Autodesk Inventor part; units mm, degrees
ref_plane "YZ Plane" through (0, 0, 0) normal (1, 0, 0) x (0, 1, 0)
ref_plane "XZ Plane" through (0, 0, 0) normal (0, 1, 0) x (-1, 0, 0)
ref_plane "XY Plane" through (0, 0, 0) normal (0, 0, 1) x (1, 0, 0)
sketch "Sketch1" plane through (0, 0, 0) normal (0, 0, 1) x (1, 0, 0)
  circle A0 centre (0, 0) radius 18
  dimension "d0" = 36
extrude "Extrusion1" add sketch "Sketch1" along normal blind 2.5
sketch "Sketch2" plane through (0, 0, 2.5) normal (0, 0, 1) x (1, 0, 0)
  line L0 (0, 0) -> (0, 11)
  circle A0 centre (0, 11) radius 1.25
  circle A1 centre (0, 0) radius 5
  circle A2 centre (7.7782, 7.7782) radius 1.25
  circle A3 centre (11, 0) radius 1.25
  circle A4 centre (7.7782, -7.7782) radius 1.25
  circle A5 centre (0, -11) radius 1.25
  circle A6 centre (-7.7782, -7.7782) radius 1.25
  circle A7 centre (-11, 0) radius 1.25
  circle A8 centre (-7.7782, 7.7782) radius 1.25
  dimension "d3" = 11
  dimension "d4" = 2.5
  dimension "d5" = 10
  dimension "d8" = 360
extrude "Extrusion2" cut sketch "Sketch2" against normal through all
sketch "Sketch3" plane through (0, 0, 2.5) normal (0, 0, 1) x (1, 0, 0)
  circle A0 centre (0, 0) radius 5.25
  dimension "d12" = 10.5
extrude "Extrusion3" cut sketch "Sketch3" against normal through all
sketch "Sketch4" plane through (0, 0, 2.5) normal (0, 0, 1) x (1, 0, 0)
  circle A0 centre (0, 11) radius 1.25
  circle A1 centre (0, 11) radius 1.35
  circle A2 centre (7.7782, 7.7782) radius 1.25
  circle A3 centre (7.7782, 7.7782) radius 1.35
  circle A4 centre (11, 0) radius 1.25
  circle A5 centre (11, 0) radius 1.35
  circle A6 centre (-7.7782, 7.7782) radius 1.25
  circle A7 centre (-7.7782, 7.7782) radius 1.35
  circle A8 centre (-11, 0) radius 1.25
  circle A9 centre (-11, 0) radius 1.35
  circle A10 centre (-7.7782, -7.7782) radius 1.25
  circle A11 centre (-7.7782, -7.7782) radius 1.35
  circle A12 centre (0, -11) radius 1.25
  circle A13 centre (0, -11) radius 1.35
  circle A14 centre (7.7782, -7.7782) radius 1.25
  circle A15 centre (7.7782, -7.7782) radius 1.35
  point P0 (0, 0)
  dimension "d15" = 2.7
  dimension "d16" = 2.7
  dimension "d17" = 2.7
  dimension "d18" = 2.7
  dimension "d19" = 2.7
  dimension "d20" = 2.7
  dimension "d21" = 2.7
  dimension "d22" = 2.7
extrude "Extrusion4" cut sketch "Sketch4" against normal blind 10
properties part number "Pulley_base"
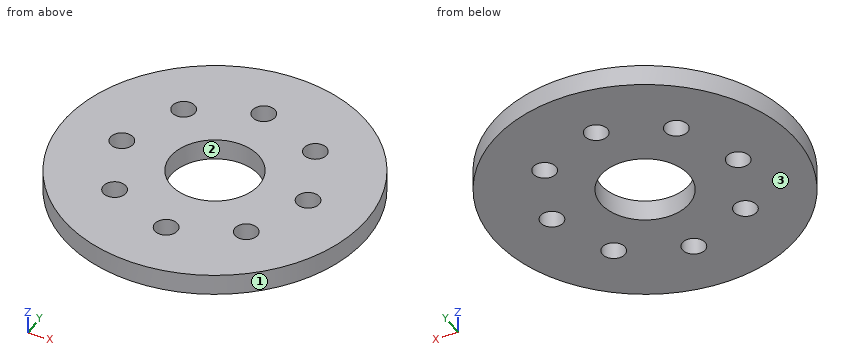
Part model, mm, in its own coordinate system. Face numbers are marked on the shaded views. Round coordinates to 2 decimals unless told otherwise and drop trailing zeros. Loops run counter-clockwise (first coordinate to the right, second up) from the corner with the lowest first, then second, coordinate; pieces in that order, holes last. Notation, with made-up numbers: (58.5, 15.25) -> (114.5, 15.25) arc R23 ccw to (114.5, 38.25) -> close; hole circle Ø8 at (-12, 7.5). An arc over 180 degrees is marked (long way). Use CSV: the item, a comma, the result in double quotes. Start each with the question number.
1) Drop flat-ended pins along their axis: P1, Ø1.5, axis at y = 5.5, z = 0.5, coming from the -X side; P2, Ø1.6, axis at x = -11, y = 0, coming from the +Z side. Give the stop position or say it passes through.
2) Cut at A-A, the plane x = 0. Write the cut outline in (y, z).
3) Cut at B-B, the plane x = 11. Write the cut outline in (y, z), plus the area to 3 significant figures.
4) Wall check: L1, parallel to Y at x = 0, z = 1.25; L2, parallel to Y at x = -9, z = 1.4; L3, parallel to X at y = -7.5, z = 2.1. Give the ranges that are in metal, low to high. Write a range as [from, to].
5) Cut at D-D, the plane z = 2.1. Give the number of separate pieces and of enclosed holes in the cut face, plus the area to 3 significant figures.
6) Pull direction X, two halves, no side cores. Call the marked faces 1, 2 and 3: +X half, -X half, draft (parallel to the pull), parting line (faces both ways), or undercut.
Determined:
1,P1,"stops at x = -17.36"
1,P2,"passes through"
2,outline,"(-18, 0) -> (-12.35, 0) -> (-12.35, 2.5) -> (-18, 2.5) -> close; (-9.65, 0) -> (-5.25, 0) -> (-5.25, 2.5) -> (-9.65, 2.5) -> close; (5.25, 0) -> (9.65, 0) -> (9.65, 2.5) -> (5.25, 2.5) -> close; (12.35, 0) -> (18, 0) -> (18, 2.5) -> (12.35, 2.5) -> close"
3,outline,"(-14.25, 0) -> (-1.35, 0) -> (-1.35, 2.5) -> (-14.25, 2.5) -> close; (1.35, 0) -> (14.25, 0) -> (14.25, 2.5) -> (1.35, 2.5) -> close"
3,area,"64.5 mm2"
4,L1,"y = [-18, -12.35], [-9.65, -5.25], [5.25, 9.65], [12.35, 18]"
4,L2,"y = [-15.59, -8.35], [-7.2, 7.2], [8.35, 15.59]"
4,L3,"x = [-16.36, -9.1], [-6.46, 6.46], [9.1, 16.36]"
5,separate pieces,"1"
5,enclosed holes,"9"
5,area,"885 mm2"
6,face 1,"parting line"
6,face 2,"undercut"
6,face 3,"draft"
